from build123d import *

# Parameters (mm, degrees)
F1_DEPTH = 282.5
F2_R     = 71
F3_DEPTH = 101.881547
F5_DEPTH = 101.881547


with BuildPart() as f1:
    # F0 (on Right) → F1 (new body, symmetric)
    with BuildSketch(Plane.YZ):
        Polygon((-23.392175, 230), (-101.880547, 80), (-99.222448, 78.609134), (-20.006297, 230), align=None)
    extrude(amount=F1_DEPTH, both=True)

    # F2 (on Front) → F3 (cut, through all)
    with BuildSketch(Plane.XZ):
        with Locations((0, 230)):
            Circle(F2_R)
    extrude(amount=F3_DEPTH, mode=Mode.SUBTRACT)

    # F4 (on Front) → F5 (cut, through all)
    with BuildSketch(Plane.XZ):
        Polygon((408.706428, 306.349989), (69.978568, 306.349989), (69.289558, 306.349989), (69.289558, 271.222025), (69.289558, 214.509451), (275.742, 17.306537), (275.742, 0), (282.5, 0), (408.706428, 0), align=None)
        Polygon((-69.289558, 271.222025), (-69.289558, 306.349989), (-69.978568, 306.349989), (-408.706428, 306.349989), (-408.706428, 0), (-282.5, 0), (-275.742, 0), (-275.742, 17.306537), (-69.289558, 214.509451), align=None)
    extrude(amount=F5_DEPTH, mode=Mode.SUBTRACT)


solid = f1.part
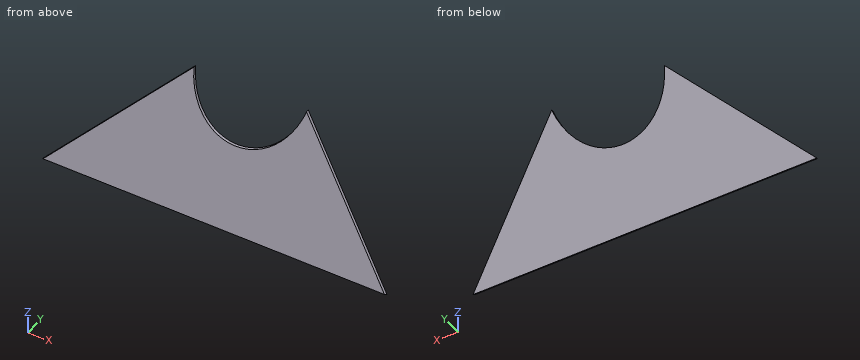
Work out the finished part from the listing and answer in its coordinate system (mm). Give positions to 0.01 mm unless a question says otherwise; leave off trailing zeros. Write each loop counter-clockwise with the first axis right and the second up, starting at its lowest first coordinate (ties: lowest second). Pieces come first, ordered by that corner, then holes.
Q1. Given pin 1 (12 mm diameter, centred on x = 135.5, y = -65, fed in from -Z); pin 2 (8 mm diameter, centred on x = -107.5, z = 157, fed in from -Y); pin 3 (3 mm diameter, centred on x = -36.5, y = -81, fed in from +Z), each flat-ended and moving along its own axis, determine where each tip first touches the part or whether it passes through.
Answer:
pin 1: stops at z = 132.55
pin 2: stops at y = -63.68
pin 3: stops at z = 122.77
Q2. The part is cut by section D-D on z = 110.5. Give the vertices of the cut face in (x, y), and give its area (3 significant figures).
Answer:
outline: (-178.18, -85.92) - (178.18, -85.92) - (178.18, -82.54) - (-178.18, -82.54) - close
area: 1,210 mm2
Q3. The part is cut by section A-A on y = -43. Give the vertices of the cut face in (x, z).
Answer:
outline: (-99.08, 186.06) - (-55.77, 186.06) arc R71 cw to (-60.31, 192.53) - (-92.3, 192.53) - close; (55.77, 186.06) - (99.08, 186.06) - (92.3, 192.53) - (60.31, 192.53) arc R71 cw to start
Q4. The part is cut by section C-C on x = 97.5. Give the vertices of the cut face in (y, z).
Answer:
outline: (-101.88, 80) - (-99.22, 78.61) - (-42.21, 187.56) - (-45.6, 187.56) - close
Q5. The part is cut by section B-B on z = 183. Give the vertices of the cut face in (x, y), and give its area (3 significant figures).
Answer:
outline: (-102.28, -47.99) - (-53.22, -47.99) - (-53.22, -44.6) - (-102.28, -44.6) - close; (53.22, -47.99) - (102.28, -47.99) - (102.28, -44.6) - (53.22, -44.6) - close
area: 332 mm2
Q6. Straight lines are drawn through the part: L1, parallel to X at y = -55, z = 168; L2, parallel to Y at x = -68, z = 159; L3, parallel to Z at x = 138.5, y = -72. For each, find the intervals that lie inside material, in ascending order.
Answer:
L1: x = -117.98 to -34.6, 34.6 to 117.98
L2: y = -60.54 to -57.16
L3: z = 130.63 to 137.11
